Autodesk Inventor part; units mm, degrees
ref_plane "YZ Plane" through (0, 0, 0) normal (1, 0, 0) x (0, 1, 0)
ref_plane "XZ Plane" through (0, 0, 0) normal (0, 1, 0) x (-1, 0, 0)
ref_plane "XY Plane" through (0, 0, 0) normal (0, 0, 1) x (1, 0, 0)
sketch "Sketch1" plane through (0, 0, 0) normal (0, 0, 1) x (1, 0, 0)
  line L0 (83, 0) -> (83, 180)
  line L1 (83, 180) -> (0, 180)
  line L2 (0, 180) -> (0, 0)
  circle A0 centre (41.5, 45) radius 15
  line L3 (0, 0) -> (83, 0)
  line L4 (10, 171.8151) -> (10, 9.9445)
  line L5 (73, 174.9264) -> (73, 13.0559)
  circle A1 centre (10, 160) radius 2
  circle A2 centre (73, 160) radius 2
  circle A3 centre (10, 20) radius 2
  circle A4 centre (73, 20) radius 2
  dimension "d0" = 83
  dimension "d1" = 180
  dimension "d4" = 30
  dimension "d5" = 41.5
  dimension "d10" = 10
  dimension "d11" = 10
  dimension "d12" = 4
  dimension "d13" = 20
  dimension "d14" = 20
  dimension "d15" = 20
  dimension "d16" = 20
  dimension "d17" = 4
  dimension "d18" = 4
  dimension "d19" = 4
extrude "Extrusion1" add sketch "Sketch1" along normal blind 3
equation "\"d5\" = 0.5 * d0"
equation "\"d11\" = d10"
equation "\"d14\" = d13"
equation "\"d15\" = d13"
equation "\"d16\" = d13"
equation "\"d17\" = d12"
equation "\"d18\" = d12"
equation "\"d19\" = d18"
equation "\"d6\" = 0.25 * d1"
properties part number "BaseC_3" material "PMMA Plastic"
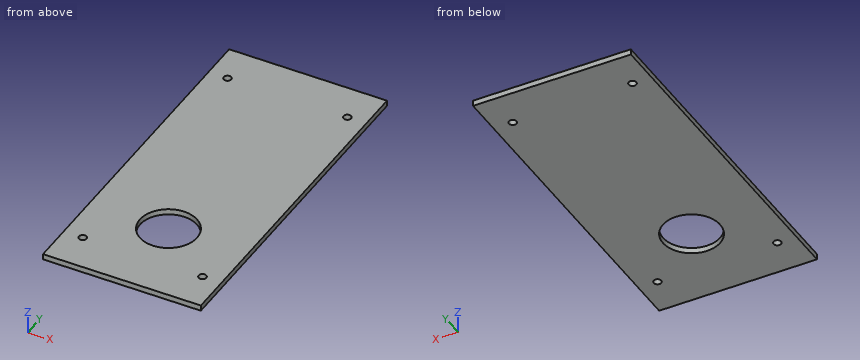
The listing builds one solid part. Answer for the finished solid, in the listing's coordinates (mm). Give positions to 0.01 mm unless a question says otherwise; leave off trailing zeros. Write each loop counter-clockwise with the first axis right and the second up, starting at its lowest first coordinate (ties: lowest second). Pieces come first, ordered by that corner, then holes.
1) Section B-B (x = 41.5) is taken. Write down the section's boundary in (y, z), and give its area (3 significant figures).
2) Find the intervals of material crossed by L1, parallel to X at y = 160, z = 1.95; L2, parallel to Y at x = 73, z = 1.55; L3, parallel to Y at x = 41.5, z = 1.9, in increasing order.
3) Section C-C (y = 45) is taken. Write down the section's boundary in (x, z).
4) Section A-A (y = 20) is taken. Write down the section's boundary in (x, z).
5) Section D-D (x = 73) is taken. Write down the section's boundary in (y, z).
Response:
1. outline: (0, 0) - (30, 0) - (30, 3) - (0, 3) - close; (60, 0) - (180, 0) - (180, 3) - (60, 3) - close
1. area: 450 mm2
2. L1: x = 0 to 8, 12 to 71, 75 to 83
2. L2: y = 0 to 18, 22 to 158, 162 to 180
2. L3: y = 0 to 30, 60 to 180
3. outline: (0, 0) - (26.5, 0) - (26.5, 3) - (0, 3) - close; (56.5, 0) - (83, 0) - (83, 3) - (56.5, 3) - close
4. outline: (0, 0) - (8, 0) - (8, 3) - (0, 3) - close; (12, 0) - (71, 0) - (71, 3) - (12, 3) - close; (75, 0) - (83, 0) - (83, 3) - (75, 3) - close
5. outline: (0, 0) - (18, 0) - (18, 3) - (0, 3) - close; (22, 0) - (158, 0) - (158, 3) - (22, 3) - close; (162, 0) - (180, 0) - (180, 3) - (162, 3) - close
